Here's how the part is built. I have some questions about the finished solid (model axes, mm). A direction names the side the tool comes from. Coordinates: 2 decimals unless noted, no trailing zeros. Write each loop counter-clockwise with the first axis right and the second up, starting at its lowest first coordinate (ties: lowest second). Pieces come first, ordered by that corner, then holes. Notation, with made-up numbers: (87, 48.5) -> (107, 48.5) arc R12 ccw to (107, 54.5) -> close; hole circle Ø2 at (41.25, 25.25). An arc over 180 degrees is marked (long way). Use CSV: the item, a comma, the result in double quotes. Start each with the question number.
```python
from build123d import *

# Parameters (mm, degrees)
F1_DEPTH         = 406.4
F2_R             = 38.1
F3_DEPTH         = 387.351
F4_R             = 38.1
F5_DEPTH         = 387.351
F8_W             = 139.2440905122
F8_H             = 374.65
F9_DEPTH         = 336.5510000866
F10_W            = 139.2440905122
F10_H            = 374.65
F11_DEPTH        = 336.551
F12_R            = 50.8
F13_DEPTH        = 406.401
F15_W            = 112.3258540089
F15_H            = 374.65
F16_DEPTH        = 215.901
F19_D            = 11.50874
F19_DEPTH        = 54.61
F19_TIP          = 3.4575743203
F19_ON_F17_D     = 11.50874
F19_ON_F17_DEPTH = 54.61
F19_ON_F17_TIP   = 3.4575743203


with BuildPart() as f1:
    # F0 (on Front) → F1 (new body)
    with BuildSketch(Plane.XZ):
        Polygon((-67.8147737194, 29.4704525612), (-215.9, -56.0265926949), (-101.6, -254), (101.6, -254), (215.9, -56.0265926949), (67.8147737194, 29.4704525612), (50.8, 0), (-50.8, 0), align=None)
    extrude(amount=F1_DEPTH)

    # F2 (on face) → F3 (cut, through all)
    with BuildSketch(Plane(origin=(29.7147737194, 0, 51.4674978174), x_dir=(0.8660254038, 0, -0.5), z_dir=(0.5, 0, 0.8660254038))):
        with Locations((129.4911357684, -76.2)):
            Circle(F2_R)
        with Locations((129.4911357684, -165.1)):
            Circle(F2_R)
        with Locations((129.4911357684, -254)):
            Circle(F2_R)
        with Locations((129.4911357684, -342.9)):
            Circle(F2_R)
    extrude(amount=-F3_DEPTH, mode=Mode.SUBTRACT)

    # F4 (on face) → F5 (cut, through all)
    with BuildSketch(Plane(origin=(-29.7147737194, 0, 51.4674978174), x_dir=(0.8660254038, 0, 0.5), z_dir=(-0.5, 0, 0.8660254038))):
        with Locations((-129.4911357684, -63.5)):
            Circle(F4_R)
        with Locations((-129.4911357684, -152.4)):
            Circle(F4_R)
        with Locations((-129.4911357684, -241.3)):
            Circle(F4_R)
        with Locations((-129.4911357684, -330.2)):
            Circle(F4_R)
    extrude(amount=-F5_DEPTH, mode=Mode.SUBTRACT)

    # F8 (on offset) → F9 (cut, through all)
    with BuildSketch(Plane(origin=(4.3147737194, 0, 7.4734073051), x_dir=(0.8660254038, 0, -0.5), z_dir=(0.5, 0, 0.8660254038))):
        with Locations((129.4911357684, -203.2)):
            Rectangle(F8_W, F8_H)
    extrude(amount=-F9_DEPTH, mode=Mode.SUBTRACT)

    # F10 (on offset) → F11 (cut, through all)
    with BuildSketch(Plane(origin=(-4.3147737194, 0, 7.4734073051), x_dir=(0.8660254038, 0, 0.5), z_dir=(-0.5, 0, 0.8660254038))):
        with Locations((-129.4911357684, -203.2)):
            Rectangle(F10_W, F10_H)
    extrude(amount=-F11_DEPTH, mode=Mode.SUBTRACT)

    # F12 (on face) → F13 (cut, through all)
    with BuildSketch(Plane.XZ.offset(406.4)):
        with Locations((0, -258.9822715367)):
            Circle(F12_R)
    extrude(amount=-F13_DEPTH, mode=Mode.SUBTRACT)

    # F15 (on offset) → F16 (cut, through all)
    with BuildSketch(Plane.XY.offset(-38.1)):
        with Locations((0, -203.2)):
            Rectangle(F15_W, F15_H)
    extrude(amount=-F16_DEPTH, mode=Mode.SUBTRACT)

    # F19
    with Locations(Plane(origin=(-29.7147737194, 0, 51.4674978174), x_dir=(0.8660254038, 0, 0.5), z_dir=(-0.5, 0, 0.8660254038))):
        with Locations((-195.9381810245, -381), (-63.0440905122, -381), (-63.0440905122, -292.1), (-195.9381810245, -292.1), (-195.9381810245, -203.2), (-63.0440905122, -203.2), (-63.0440905122, -114.3), (-195.9381810245, -114.3), (-195.9381810245, -25.4), (-63.0440905122, -25.4)):
            Hole(F19_D / 2, depth=F19_DEPTH)
            with Locations((0, 0, -(F19_DEPTH + F19_TIP / 2))):  # 118° drill point
                Cone(0, F19_D / 2, F19_TIP, mode=Mode.SUBTRACT)

    # F19 on F17
    with Locations(Plane(origin=(29.7147737194, 0, 51.4674978174), x_dir=(0.8660254038, 0, -0.5), z_dir=(0.5, 0, 0.8660254038))):
        with Locations((63.0440905122, -25.4), (63.0440905122, -114.3), (63.0440905122, -203.2), (63.0440905122, -292.1), (63.0440905122, -381), (195.9381810245, -381), (195.9381810245, -292.1), (195.9381810245, -203.2), (195.9381810245, -114.3), (195.9381810245, -25.4)):
            Hole(F19_ON_F17_D / 2, depth=F19_ON_F17_DEPTH)
            with Locations((0, 0, -(F19_ON_F17_DEPTH + F19_ON_F17_TIP / 2))):  # 118° drill point
                Cone(0, F19_ON_F17_D / 2, F19_ON_F17_TIP, mode=Mode.SUBTRACT)


solid = f1.part
```
Item 1: I want a section at D-D on z = -122.5. Please give me the cut outline in (x, y) (3 decimals).
Item 2: I want a section at B-B on z = -223.5. Please give me the cut outline in (x, y) (3 decimals).
Item 3: Which directions (+Z, -Z, +X, -X, +Y, -Y) give clear straight access to the entire face, cutting with the end or side of a thin tool? Please do faces 4 (the flat face through (-159.55, -200.36, -153.63)), 5 (the flat face through (-1, -201, -38.1)), 6 (the flat face through (5, -390.525, -147)).
Item 4: Thinking about a two-plate mould opening in X: for faces 1 (the flat face through (51.71, -205.82, -30.17)), 2 (the flat face through (-140.82, -200.36, -12.68)), 3 (the flat face through (159.348, -200.355, -23.376)), which applies, +X half, -X half, draft (parallel to the pull), parting line (faces both ways), or undercut?
Item 5: If I drill on line 1 along Y through (x, z) = (5, -187) (3 decimals); line 2 along Y through (x, z) = (168.5, -30); line 3 along Y through (x, z) = (161.5, -47), over which ranges is the centre line in solid material (lowest first)?
Item 6: I want a section at C-C on x = 122.5. Count the separate pieces of the cut face and the enclosed holes in it, then the cut area to 3 significant figures.
Item 7: I'm going to push flat-ended pins straight in: pin 1 (2 mm diameter, centred on x = -83, z = -55.5, fed in from +Y); pin 2 (2 mm diameter, centred on y = -57, z = -12, fed in from +X); pin 3 (2 mm diameter, centred on y = -246, z = -84.5, fed in from +X); pin 4 (1.5 mm diameter, centred on x = 57, y = -170.5, fed in from +Z). Where does each tip first touch, or does it pass through?
Item 8: I want a section at A-A on y = -235. Please give me the cut outline in (x, z), then the cut area to 3 significant figures.
Geometry says:
1,outline,"(-177.522, -406.4) -> (177.522, -406.4) -> (177.522, 0) -> (-177.522, 0) -> close; hole (-159.191, -390.525) -> (159.191, -390.525) -> (159.191, -15.875) -> (-159.191, -15.875) -> close"
2,outline,"(-119.209, -406.4) -> (-36.354, -406.4) -> (-36.354, -390.525) -> (-100.878, -390.525) -> (-100.878, -15.875) -> (-36.354, -15.875) -> (-36.354, 0) -> (-119.209, 0) -> close; (36.354, -406.4) -> (119.209, -406.4) -> (119.209, 0) -> (36.354, 0) -> (36.354, -15.875) -> (100.878, -15.875) -> (100.878, -390.525) -> (36.354, -390.525) -> close"
3,face 4,"-Z, -X, +Y, -Y"
3,face 5,"-Z"
3,face 6,"none"
4,face 1,"undercut"
4,face 2,"-X half"
4,face 3,"+X half"
5,line 1,"-406.4 to -390.525, -15.875 to 0"
5,line 2,"-406.4 to -364.43, -321.37 to -275.53, -232.47 to -186.63, -143.57 to -97.73, -54.67 to 0"
5,line 3,"-406.4 to -360.34, -325.46 to -271.44, -236.56 to -182.54, -147.66 to -93.64, -58.76 to 0"
6,separate pieces,"4"
6,enclosed holes,"0"
6,area,"23,700 mm2"
7,pin 1,"y = 0"
7,pin 2,"x = 105.5"
7,pin 3,"x = 200.04"
7,pin 4,"z = 12.04"
8,outline,"(-215.9, -56.03) -> (-101.6, -254) -> (-83.27, -254) -> (-176.75, -92.08) -> (-149, -76.06) -> (-174.4, -32.07) -> close; (-109.32, 5.51) -> (-83.92, -38.48) -> (-56.16, -22.46) -> (-47.13, -38.1) -> (47.13, -38.1) -> (56.16, -22.46) -> (87.86, -40.76) -> (113.26, 3.23) -> (67.81, 29.47) -> (50.8, 0) -> (-50.8, 0) -> (-67.81, 29.47) -> close; (83.27, -254) -> (101.6, -254) -> (215.9, -56.03) -> (170.46, -29.79) -> (145.06, -73.78) -> (176.75, -92.08) -> close"
8,area,"19,700 mm2"
